```python
from build123d import *
from build123d.topology import SkipClean

# Parameters (mm, degrees)
CROQUIS2_R                   = 0.5
SALIENTE_EXTRUIR1_DEPTH      = 0.5
SALIENTE_EXTRUIR1_DEPTH_BACK = 0.5
CROQUIS3_R                   = 1.25
CROQUIS3_R_2                 = 0.75


with BuildPart() as part:
    # Barrer1: sweep along a path in Croquis1
    with BuildLine(Plane.XY) as barrer1_path:
        Line((0, 0), (-450, 0))
    # Croquis2 → Barrer1 (sweep)
    with BuildSketch(Plane(origin=(0, 0, 0), x_dir=(0, 0, -1), z_dir=(1, 0, 0))):
        Circle(CROQUIS2_R)
    sweep(path=barrer1_path.line)

    # Croquis3 → Saliente-Extruir1 (add, two sides: drawn at the far end of the back side and taken through both)
    # profile 1 of 2: a face of its own
    with SkipClean():  # the faces are left unmerged after this step: merging them gives an invalid solid
        with BuildSketch(Plane.XY.offset(-SALIENTE_EXTRUIR1_DEPTH_BACK)):
            with Locations((1, 0)):
                Circle(CROQUIS3_R)
            with Locations((1, 0)):
                Circle(CROQUIS3_R_2, mode=Mode.SUBTRACT)
        # profile 2 of 2: a face of its own
        with BuildSketch(Plane.XY.offset(-SALIENTE_EXTRUIR1_DEPTH_BACK)):
            with Locations((-451, 0)):
                Circle(CROQUIS3_R)
            with Locations((-451, 0)):
                Circle(CROQUIS3_R_2, mode=Mode.SUBTRACT)
        extrude(amount=SALIENTE_EXTRUIR1_DEPTH + SALIENTE_EXTRUIR1_DEPTH_BACK)


solid = part.part
```
Verification items for the finished model (mm, model axes). Give positions to 0.01 mm unless a question says otherwise; leave off trailing zeros. Loops run counter-clockwise (first coordinate to the right, second up) from the corner with the lowest first, then second, coordinate; pieces in that order, holes last.
1. Thickness scan on line 1 (X direction, y = -0.05, z = -0.15); line 2 (X direction, y = -1, z = -0.3); line 3 (Y direction, x = 1, z = 0.2). Record the ranges inside material, lowest first.
2. Section check B-B, the plane x = -340. Enter the section's corners in (y, z), then the cut area to 3 significant figures.
3. Section check A-A, the plane z = 0. Enter the section's corners in (x, y), then the cut area to 3 significant figures.
Geometry says:
1. line 1: x = -452.25 to -451.75, -450.25 to 0.25, 1.75 to 2.25
1. line 2: x = -451.75 to -450.25, 0.25 to 1.75
1. line 3: y = -1.25 to -0.75, 0.75 to 1.25
2. outline: circle Ø1 at (0, 0)
2. area: 0.785 mm2
3. outline: (-449.85, -0.5) - (-0.15, -0.5) arc R1.25 ccw (long way) to (-0.15, 0.5) - (-449.85, 0.5) arc R1.25 ccw (long way) to start; hole circle Ø1.5 at (-451, 0); hole circle Ø1.5 at (1, 0)
3. area: 456 mm2
